Can you work these out from the model? Positions are in its coordinate system, mm. A direction names the side the tool comes from. Give positions to 0.01 mm unless a question says otherwise; leave off trailing zeros. Loops run counter-clockwise (first coordinate to the right, second up) from the corner with the lowest first, then second, coordinate; pieces in that order, holes last. Notation, with made-up numbers: M 34,-37.5 L 63,-37.5 A3 cw 63,-33.5 Z; hole C 52,77.25 d5. An arc over 180 degrees is marked long. Answer as a JSON object with one key per item and string values.
```python
from build123d import *

# Parameters (mm, degrees)
BOSS_EXTRUDE1_DEPTH = 6.5
SKETCH2_W           = 60.158889846
SKETCH2_H           = 160
BOSS_EXTRUDE3_DEPTH = 5
SKETCH6_R           = 3
CUT_EXTRUDE7_DEPTH  = 5.1
BOSS_EXTRUDE4_DEPTH = 31
CUT_EXTRUDE8_REACH  = 196.785
SKETCH11_W          = 5.5
SKETCH11_H          = 10.5
CUT_EXTRUDE9_REACH  = 194.771
SKETCH13_R          = 1.5
CUT_EXTRUDE10_DEPTH = 17
CUT_EXTRUDE11_REACH = 196.785
SKETCH14_R          = 3
BOSS_EXTRUDE5_START = -5
SKETCH15_R          = 1.5
BOSS_EXTRUDE5_DEPTH = 5
RIB2_START          = -2.5
RIB2_DEPTH          = 5
CUT_EXTRUDE12_REACH = 196.785
SKETCH17_W          = 8
SKETCH17_H          = 13
FILLET1_R           = 4
FILLET2_R           = 0.5
SWEEP1_PROFILE_R    = 2.5


# Read off the part's stored shape, not the designer's step: Rib2
with BuildPart() as part:
    # Sketch1 → Boss-Extrude1 (new body)
    with BuildSketch(Plane.XY):
        with BuildLine():
            Line((-15.5, -70), (-15.5, 30))
            Line((-15.5, 30), (15.5, 30))
            Line((15.5, 30), (15.5, -70))
            add(Edge.make_bspline(
                [(15.5, -70), (15.682751911, -79.304401058), (30, -150)],
                knots=[0.243669215, 0.243669215, 0.243669215, 1, 1, 1], degree=2))
            Line((30, -150), (-30, -150))
            add(Edge.make_bspline(
                [(-15.5, -70), (-15.682751911, -79.304401058), (-30, -150)],
                knots=[0.243669215, 0.243669215, 0.243669215, 1, 1, 1], degree=2))
        make_face()
    extrude(amount=BOSS_EXTRUDE1_DEPTH)

    # Sketch2 → Boss-Extrude3 (add)
    with BuildSketch(Plane(origin=(0, -75, -75), x_dir=(1, 0, 0), z_dir=(0, 0.7071067811865488, 0.7071067811865464))):
        with Locations((0.079444923, -30.662211256)):
            Rectangle(SKETCH2_W, SKETCH2_H)
    extrude(amount=BOSS_EXTRUDE3_DEPTH)

    # Sketch6 → Cut-Extrude7 (cut)
    with BuildSketch(Plane(origin=(0, -75, -75), x_dir=(-1, 0, 0), z_dir=(0, -0.7071067811865487, -0.7071067811865464))):
        with Locations(Location((-20.158889846, -20.363007156, 0), (0, 0, 90))):
            Circle(SKETCH6_R)
        with Locations(Location((20, -20.363007156, 0), (0, 0, 90))):
            Circle(SKETCH6_R)
        with Locations(Location((-0.079444923, 39.337788744, 0), (0, 0, 90))):
            Circle(SKETCH6_R)
    extrude(amount=-CUT_EXTRUDE7_DEPTH, mode=Mode.SUBTRACT)

    # Sketch10 → Boss-Extrude4 (add)
    with BuildSketch(Plane(origin=(15.5, 0, 0), x_dir=(0, 0, -1), z_dir=(1, 0, 0))):
        with BuildLine():
            Line((-6.5, 36.5), (-6.5, 30))
            Line((-6.5, 30), (0, 30))
            ThreePointArc((0, 30), (-1.903805922, 34.596194078), (-6.5, 36.5))
        make_face()
    extrude(amount=-BOSS_EXTRUDE4_DEPTH)

    # Sketch11 → Cut-Extrude8 (cut, up to next)
    with BuildSketch(Plane.XY.offset(6.5), mode=Mode.PRIVATE) as cut_extrude8_sk1:
        with Locations((12.75, 31.25)):
            Rectangle(SKETCH11_W, SKETCH11_H)
    cut_extrude8_tool1 = extrude(cut_extrude8_sk1.sketch, amount=-CUT_EXTRUDE8_REACH, mode=Mode.PRIVATE) & part.part
    add(cut_extrude8_tool1.solids().sort_by_distance((12.75, 31.25, 6.5))[0], mode=Mode.SUBTRACT)

    # Sketch12 → Cut-Extrude9 (cut, up to next)
    with BuildSketch(Plane(origin=(10, 0, 0), x_dir=(0, 0, -1), z_dir=(1, 0, 0)), mode=Mode.PRIVATE) as cut_extrude9_sk1:
        with BuildLine():
            Line((-6.5, 34), (-6.5, 26))
            ThreePointArc((-6.5, 26), (-2.5, 30), (-6.5, 34))
        make_face()
    cut_extrude9_tool1 = extrude(cut_extrude9_sk1.sketch, amount=-CUT_EXTRUDE9_REACH, mode=Mode.PRIVATE) & part.part
    add(cut_extrude9_tool1.solids().sort_by_distance((10, 30, 4.802347))[0], mode=Mode.SUBTRACT)

    # Sketch13 → Cut-Extrude10 (cut)
    with BuildSketch(Plane(origin=(-3.389594105, 24.118215268, 0), x_dir=(0, 0, 1), z_dir=(-0.13917310096006605, 0.9902680687415703, 0))):
        with Locations(Location((3, 15.121181312, 0), (0, 0, 270))):
            Circle(SKETCH13_R)
    extrude(amount=-CUT_EXTRUDE10_DEPTH, mode=Mode.SUBTRACT)

    # Sketch14 → Cut-Extrude11 (cut, up to next)
    with BuildSketch(Plane.XY.offset(6.5), mode=Mode.PRIVATE) as cut_extrude11_sk1:
        with Locations((5.5, 16.5)):
            Circle(SKETCH14_R)
    cut_extrude11_tool1 = extrude(cut_extrude11_sk1.sketch, amount=-CUT_EXTRUDE11_REACH, mode=Mode.PRIVATE) & part.part
    # Sketch14 → Cut-Extrude11 (cut, up to next)
    with BuildSketch(Plane.XY.offset(6.5), mode=Mode.PRIVATE) as cut_extrude11_sk2:
        with Locations((5.5, -5)):
            Circle(SKETCH14_R)
    cut_extrude11_tool2 = extrude(cut_extrude11_sk2.sketch, amount=-CUT_EXTRUDE11_REACH, mode=Mode.PRIVATE) & part.part
    add(cut_extrude11_tool1.solids().sort_by_distance((5.5, 16.5, 6.5))[0], mode=Mode.SUBTRACT)
    add(cut_extrude11_tool2.solids().sort_by_distance((5.5, -5, 6.5))[0], mode=Mode.SUBTRACT)

    # Sketch15 → Boss-Extrude5 (add)
    with BuildSketch(Plane.ZY.offset(30).offset(BOSS_EXTRUDE5_START)):
        with BuildLine():
            Line((2.923559779, 35.427621518), (-106.351551084, -36.577381104))
            Line((-106.351551084, -36.577381104), (-60.077932214, -82.850999974))
            Line((-60.077932214, -82.850999974), (10.840158065, 25.161298937))
            ThreePointArc((10.840158065, 25.161298937), (11.647345051, 33.969236568), (2.923559779, 35.427621518))
        make_face()
        with Locations(Location((6.5, 30, 0), (0, 0, 270))):
            Circle(SKETCH15_R, mode=Mode.SUBTRACT)
    extrude(amount=BOSS_EXTRUDE5_DEPTH)

    # Rib2 outline → Rib2 (add)
    with BuildSketch(Plane(origin=(-5.5, 0, 0), x_dir=(0, 0, -1), z_dir=(1, 0, 0)).offset(RIB2_START)):
        with BuildLine():
            Line((0, -142.928932188), (88.904911914, -54.024020274))
            add(Edge.make_bspline(
                [(88.904911914, -54.024020274), (20.400745035, -61.458454661), (0, -7.927359395)],
                knots=[0, 0, 0, 1, 1, 1], degree=2))
            Line((0, -7.927359395), (0, -142.928932188))
        make_face()
    extrude(amount=RIB2_DEPTH)

    # Sketch17 → Cut-Extrude12 (cut, up to next)
    with BuildSketch(Plane.XY.offset(6.5), mode=Mode.PRIVATE) as cut_extrude12_sk1:
        with Locations((-11.5, 9.5)):
            Rectangle(SKETCH17_W, SKETCH17_H)
    cut_extrude12_tool1 = extrude(cut_extrude12_sk1.sketch, amount=-CUT_EXTRUDE12_REACH, mode=Mode.PRIVATE) & part.part
    add(cut_extrude12_tool1.solids().sort_by_distance((-11.5, 9.5, 6.5))[0], mode=Mode.SUBTRACT)

    # Fillet1
    fillet1_edges = [part.edges().sort_by_distance(p)[0] for p in [
        (-15.5, 3, 3.25),
        (-15.5, 16, 3.25),
    ]]
    fillet(fillet1_edges, radius=FILLET1_R)

    # Fillet2
    fillet2_edges = [part.edges().sort_by_distance(p)[0] for p in [
        (-7.5, 16, 3.25),
        (-7.5, 3, 3.25),
    ]]
    fillet(fillet2_edges, radius=FILLET2_R)

    # Sweep1: sweep along a path in Sketch18
    with BuildLine(Plane(origin=(0, -76.482233047, 76.482233047), x_dir=(-1, 0, 0), z_dir=(0, -0.7071067811865464, 0.7071067811865488))) as sweep1_path:
        Line((27.5, 101.066017178), (27.5, 86.066017178))
        ThreePointArc((27.5, 86.066017178), (20.75, 79.316017178), (14, 86.066017178))
        Line((14, 86.066017178), (14, 101.066017178))
    # Sweep1 profile (on start of the path) → Sweep1 (sweep)
    with BuildSketch(Plane(origin=(-27.5, -147.946699141, 5.017766953), x_dir=(0, -0.7071067811865464, 0.7071067811865488), z_dir=(0, 0.7071067811865488, 0.7071067811865464))):
        Circle(SWEEP1_PROFILE_R)
    sweep(path=sweep1_path.line)


solid = part.part
```
1) For faces 4 (the flat face through (15.5, -21, 3)), 5 (the flat face through (-25, -18, -47)), 6 (the flat face through (13.3, 26, 3.3)), 7 (the flat face through (-7.5, 9, 3)), which set-ups out of +Z, -Z, +X, -X, +Y, -Y let a thin tool reach every point of the face, with its end or its side?
Answer list:
{"face 4": "+Z, +X, +Y", "face 5": "+Z, +Y", "face 6": "+Z, -Z, +X, +Y", "face 7": "+Z, -Z"}
2) Will these pins go through, and if not, where does the flat tip stop? pin 1 Ø3 at (y, z) = (-8.5, 3.5) entering from +X; pin 2 Ø7 at (x, y) = (5.5, -5) entering from -Z; pin 3 Ø3 at (x, z) = (23.5, -50) entering from +Y; pin 4 Ø4 at (y, z) = (30, 6.5) entering from -X.
Answer list:
{"pin 1": "x = 15.5", "pin 2": "z = 0", "pin 3": "y = -91.43", "pin 4": "x = -30"}
3) Please list where these lines run through material, in increasing order: line 1 along Y through (x, z) = (5, 3); line 2 along X through (y, z) = (-86, -58.5); line 3 along X through (y, z) = (-56, -77). Write a range as from..to.
Answer list:
{"line 1": "-153..-7.96, -2.04..13.54, 19.46..28.06, 31.94..35.48", "line 2": "-30..-22.86, -17.14..17.3, 23.02..30.16", "line 3": "-30..-25, -8..-3"}
4) If we mould it in two halves opening along Z, with no side actions, what happens to faces 1 (the cylindrical face through (-2.572, 34.545, 1.854)), 2 (the flat face through (-8, -74, -24)), 3 (the cylindrical face through (5.109, -2.026, 3.296))? For each: +Z half, -Z half, draft (parallel to the pull), parting line (faces both ways), or undercut.
Answer list:
{"face 1": "-Z half", "face 2": "undercut", "face 3": "draft"}
5) Suppose I cut it at A-A, the plane y = -5. Write out the boundary of the cut face in (x, z), and give its area (3 significant figures).
Answer list:
{"outline": "M -30,-58.43 L -25,-58.43 L -25,-8.96 L -30,-8.96 Z; M -15.5,0 L 2.5,0 L 2.5,6.5 L -15.5,6.5 Z; M 8.5,0 L 15.5,0 L 15.5,6.5 L 8.5,6.5 Z", "area": "410 mm^2"}
